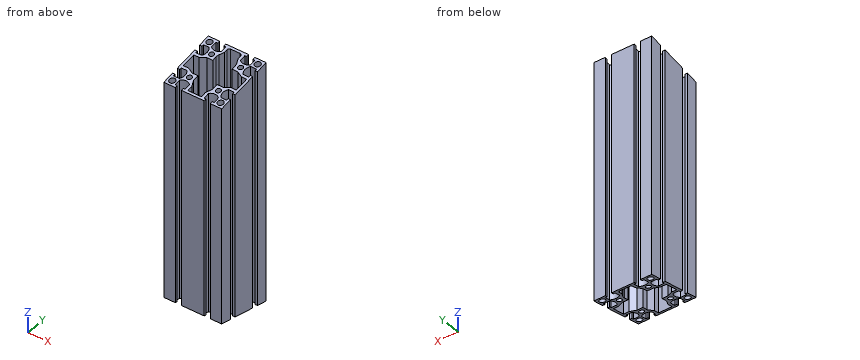
```python
from build123d import *

# Parameters (mm, degrees)
F0_R          = 3
F0_R_2        = 2.5
F1_DEPTH      = 244.595
F2_R          = 2
F3_R          = 7
F5_DEPTH      = 30
F5_DEPTH_BACK = 30


# Not quite as in the source:
# - a feature names something its author has since deleted; it is built from what else it names


with BuildPart() as f1:
    # F0 (on Top) → F1 (new body)
    with BuildSketch(Plane.XY):
        with BuildLine():
            Line((18.15, -30), (30, -30))
            Line((30, -30), (30, -18.15))
            Line((30, -18.15), (27.5, -18.15))
            Line((27.5, -18.15), (27.5, -20.15))
            Line((27.5, -20.15), (21.5477069044, -20.15))
            ThreePointArc((21.5477069044, -20.15), (19.5, -15), (21.5477069044, -9.85))
            Line((21.5477069044, -9.85), (27.5, -9.85))
            Line((27.5, -9.85), (27.5, -11.85))
            Line((27.5, -11.85), (30, -11.85))
            Line((30, -11.85), (30, 11.85))
            Line((30, 11.85), (27.5, 11.85))
            Line((27.5, 11.85), (27.5, 9.85))
            Line((27.5, 9.85), (21.5477069044, 9.85))
            ThreePointArc((21.5477069044, 9.85), (19.5, 15), (21.5477069044, 20.15))
            Line((21.5477069044, 20.15), (27.5, 20.15))
            Line((27.5, 20.15), (27.5, 18.15))
            Line((27.5, 18.15), (30, 18.15))
            Line((30, 18.15), (30, 30))
            Line((30, 30), (18.15, 30))
            Line((18.15, 30), (18.15, 27.5))
            Line((18.15, 27.5), (20.15, 27.5))
            Line((20.15, 27.5), (20.15, 21.5477069044))
            ThreePointArc((20.15, 21.5477069044), (15, 19.5), (9.85, 21.5477069044))
            Line((9.85, 21.5477069044), (9.85, 27.5))
            Line((9.85, 27.5), (11.85, 27.5))
            Line((11.85, 27.5), (11.85, 30))
            Line((11.85, 30), (-11.85, 30))
            Line((-11.85, 30), (-11.85, 27.5))
            Line((-11.85, 27.5), (-9.85, 27.5))
            Line((-9.85, 27.5), (-9.85, 21.5477069044))
            ThreePointArc((-9.85, 21.5477069044), (-15, 19.5), (-20.15, 21.5477069044))
            Line((-20.15, 21.5477069044), (-20.15, 27.5))
            Line((-20.15, 27.5), (-18.15, 27.5))
            Line((-18.15, 27.5), (-18.15, 30))
            Line((-18.15, 30), (-30, 30))
            Line((-30, 30), (-30, 18.15))
            Line((-30, 18.15), (-27.5, 18.15))
            Line((-27.5, 18.15), (-27.5, 20.15))
            Line((-27.5, 20.15), (-21.5477069044, 20.15))
            ThreePointArc((-21.5477069044, 20.15), (-19.5, 15), (-21.5477069044, 9.85))
            Line((-21.5477069044, 9.85), (-27.5, 9.85))
            Line((-27.5, 9.85), (-27.5, 11.85))
            Line((-27.5, 11.85), (-30, 11.85))
            Line((-30, 11.85), (-30, -11.85))
            Line((-30, -11.85), (-27.5, -11.85))
            Line((-27.5, -11.85), (-27.5, -9.85))
            Line((-27.5, -9.85), (-21.5477069044, -9.85))
            ThreePointArc((-21.5477069044, -9.85), (-19.5, -15), (-21.5477069044, -20.15))
            Line((-21.5477069044, -20.15), (-27.5, -20.15))
            Line((-27.5, -20.15), (-27.5, -18.15))
            Line((-27.5, -18.15), (-30, -18.15))
            Line((-30, -18.15), (-30, -30))
            Line((-30, -30), (-18.15, -30))
            Line((-18.15, -30), (-18.15, -27.5))
            Line((-18.15, -27.5), (-20.15, -27.5))
            Line((-20.15, -27.5), (-20.15, -21.5477069044))
            ThreePointArc((-20.15, -21.5477069044), (-15, -19.5), (-9.85, -21.5477069044))
            Line((-9.85, -21.5477069044), (-9.85, -27.5))
            Line((-9.85, -27.5), (-11.85, -27.5))
            Line((-11.85, -27.5), (-11.85, -30))
            Line((-11.85, -30), (11.85, -30))
            Line((11.85, -30), (11.85, -27.5))
            Line((11.85, -27.5), (9.85, -27.5))
            Line((9.85, -27.5), (9.85, -21.5477069044))
            ThreePointArc((9.85, -21.5477069044), (15, -19.5), (20.15, -21.5477069044))
            Line((20.15, -21.5477069044), (20.15, -27.5))
            Line((20.15, -27.5), (18.15, -27.5))
            Line((18.15, -27.5), (18.15, -30))
        make_face()
        with Locations((-25, -25)):
            Circle(F0_R, mode=Mode.SUBTRACT)
        with Locations((-15, -15)):
            Circle(F0_R_2, mode=Mode.SUBTRACT)
        with Locations((25, -25)):
            Circle(F0_R, mode=Mode.SUBTRACT)
        with Locations((15, -15)):
            Circle(F0_R_2, mode=Mode.SUBTRACT)
        with Locations((-25, 25)):
            Circle(F0_R, mode=Mode.SUBTRACT)
        with Locations((-15, 15)):
            Circle(F0_R_2, mode=Mode.SUBTRACT)
        Polygon((-7, 22), (-7, 27.5), (0, 27.5), (7, 27.5), (7, 22), (10, 16), (10, 10), (16, 10), (22, 7), (27.5, 7), (27.5, 0), (27.5, -7), (22, -7), (16, -10), (10, -10), (10, -16), (7, -22), (7, -27.5), (0, -27.5), (-7, -27.5), (-7, -22), (-10, -16), (-10, -10), (-16, -10), (-22, -7), (-27.5, -7), (-27.5, 0), (-27.5, 7), (-22, 7), (-16, 10), (-10, 10), (-10, 16), align=None, mode=Mode.SUBTRACT)
        with Locations((15, 15)):
            Circle(F0_R_2, mode=Mode.SUBTRACT)
        with Locations((25, 25)):
            Circle(F0_R, mode=Mode.SUBTRACT)
    extrude(amount=F1_DEPTH)

    # F2
    f2_edges = [f1.edges().sort_by_distance(p)[0] for p in [
        (-7, 27.5, 122.2975),
        (7, 27.5, 122.2975),
    ]]
    fillet(f2_edges, radius=F2_R)

    # F3
    f3_edges = [f1.edges().sort_by_distance(p)[0] for p in [
        (-10, 16, 122.2975),
        (10, 16, 122.2975),
    ]]
    fillet(f3_edges, radius=F3_R)

    # F4 (on Right) → F5 (cut, two sides)
    with BuildSketch(Plane.YZ) as f5_sk:
        Polygon((6.0593712047, -120.3576686088), (30, 0), (-94.0233882431, 24.6697857659), (-117.9640170384, -95.6878828429), align=None)
        Polygon((30, 244.595), (11.5280437604, 337.4597951001), (-122.8815300181, 310.7240685814), (-104.4095737785, 217.8592734812), align=None)
    extrude(amount=-F5_DEPTH, mode=Mode.SUBTRACT)
    extrude(f5_sk.sketch, amount=F5_DEPTH_BACK, mode=Mode.SUBTRACT)


solid = f1.part
```
Work out the finished part from the listing and answer in its coordinate system (mm). Give positions to 0.01 mm unless a question says otherwise; leave off trailing zeros. Order: outer loops, then holes, each group sorted by start corner. A loop starts at its lowest first (then second) coordinate and runs counter-clockwise, first axis right, second up.
1. Straight lines are drawn through the part: L1, parallel to Y at x = 25, z = 163; L2, parallel to X at y = 15, z = 136. For each, find the intervals that lie inside material, in ascending order.
Result sheet:
L1: y = -30 to -28, -22 to -20.15, -9.85 to -7, 7 to 9.85, 20.15 to 22, 28 to 30
L2: x = -19.5 to -17.5, -12.5 to -9.97, 9.97 to 12.5, 17.5 to 19.5
2. Section C-C, the plane y = -3 is taken. Determine the outline of the cut face in (x, z).
Result sheet:
outline: (-30, 6.56) - (-27.5, 6.56) - (-27.5, 238.03) - (-30, 238.03) - close; (27.5, 6.56) - (30, 6.56) - (30, 238.03) - (27.5, 238.03) - close
3. Section D-D, the plane z = 124 is taken. Give the number of separate pieces and of enclosed holes in the cut face, and give its area (3 significant figures).
Result sheet:
separate pieces: 1
enclosed holes: 9
area: 1,080 mm2
4. Section B-B, the plane x = 25 is taken. Determine the outline of the cut face in (y, z) (3 decimals), and give its area (3 significant figures).
Result sheet:
outline: (-30, 11.935) - (-28, 11.537) - (-28, 233.058) - (-30, 232.66) - close; (-22, 10.343) - (-20.15, 9.975) - (-20.15, 234.62) - (-22, 234.252) - close; (-9.85, 7.927) - (-7, 7.36) - (-7, 237.235) - (-9.85, 236.668) - close; (7, 4.575) - (9.85, 4.008) - (9.85, 240.587) - (7, 240.02) - close; (20.15, 1.959) - (22, 1.591) - (22, 243.004) - (20.15, 242.636) - close; (28, 0.398) - (30, 0) - (30, 244.595) - (28, 244.197) - close
area: 3,120 mm2
5. Each of these flat-tipped pins is pushed along its axis until it touches: P1, Ø10, axis at x = 13.5, y = 19, coming from the -Z side; P2, Ø5, axis at x = 20.5, y = 20.5, coming from the +Z side; P3, Ø3, axis at y = 14.5, z = 121, coming from the +X side. Where does it stop, or does it pass through?
Result sheet:
P1: stops at z = 1.51
P2: stops at z = 243.2
P3: stops at x = 19.77
6. Section A-A, the plane y = -25 is taken. Determine the outline of the cut face in (x, z), and give its area (3 significant figures).
Result sheet:
outline: (-30, 10.94) - (-28, 10.94) - (-28, 233.65) - (-30, 233.65) - close; (-22, 10.94) - (-20.15, 10.94) - (-20.15, 233.65) - (-22, 233.65) - close; (-9.85, 10.94) - (-7, 10.94) - (-7, 233.65) - (-9.85, 233.65) - close; (7, 10.94) - (9.85, 10.94) - (9.85, 233.65) - (7, 233.65) - close; (20.15, 10.94) - (22, 10.94) - (22, 233.65) - (20.15, 233.65) - close; (28, 10.94) - (30, 10.94) - (30, 233.65) - (28, 233.65) - close
area: 2,980 mm2
